CAD build for the part. Positions are in the model's coordinates, mm. Face numbers are marked on the shaded views. A direction names the side the tool comes from. Round coordinates to 2 decimals unless told otherwise and drop trailing zeros. Write each loop counter-clockwise with the first axis right and the second up, starting at its lowest first coordinate (ties: lowest second). Pieces come first, ordered by that corner, then holes. Notation, with made-up numbers: (63.5, 50.5) - (79.5, 50.5) arc R15 cw to (79.5, 63.5) - close; hole circle Ø11 at (46.5, 39). An arc over 180 degrees is marked (long way). Put each result on its own line as item: value. Start each with the question number.
Item 1: 3-axis set-ups, long thin cutter, end or side, ignore diameter. For the marked faces 1 and 2: which of +Z, -Z, +X, -X, +Y, -Y reach the whole face in a straight line?
Item 2: Cut at C-C (z = 41). Give the cut face in (x, y).
Item 3: Drill centre lines: line 1 (Z direction, x = 9.5, y = -7.75); line 2 (X direction, y = -0.25, z = 40.5); line 3 (Y direction, x = -0.5, z = 35.5). Where is each one in solid material? Low to high. Write a range as from..to.
Item 4: Cut at B-B (y = 0). Give the cut face in (x, z).
Item 5: Cut at A-A (x = 0). Give the cut face in (y, z).
Item 6: Pin check, flat tips, straight feed: pin 1 Ø5 at (x, y) = (-9.5, -0.5) entering from -Z; pin 2 Ø5 at (x, z) = (-7.5, 37) entering from +Y. Stop position of each tip, or through.
```python
from build123d import *

# Parameters (mm, degrees)
F0_W     = 29.464
F0_H     = 25.4508
F1_DEPTH = 50.9778
F2_W     = 39.90591
F2_H     = 36.580414
F2_R     = 12
F3_DEPTH = 19.05


with BuildPart() as f1:
    # F0 (on Top) → F1 (new body)
    with BuildSketch(Plane.XY):
        Rectangle(F0_W, F0_H)
    extrude(amount=F1_DEPTH)

    # F2 (on face) → F3 (cut)
    with BuildSketch(Plane.XY.offset(50.9778)):
        Rectangle(F2_W, F2_H)
        Circle(F2_R, mode=Mode.SUBTRACT)
    extrude(amount=-F3_DEPTH, mode=Mode.SUBTRACT)


solid = f1.part
```
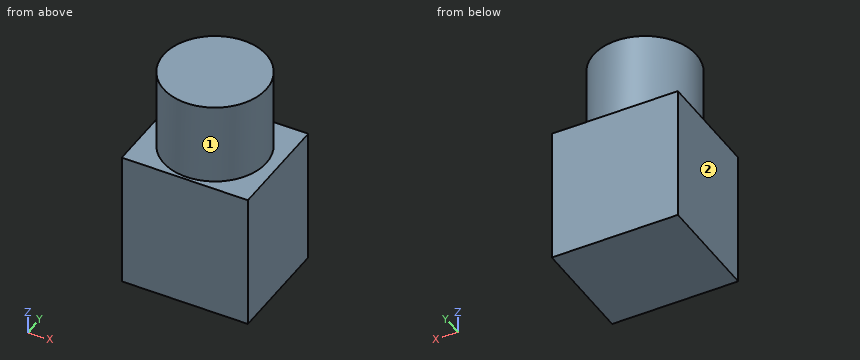
Output values:
1. face 1: +Z
1. face 2: +Z, -Z, -X, +Y, -Y
2. outline: circle Ø24 at (0, 0)
3. line 1: 0..31.93
3. line 2: -12..12
3. line 3: -11.99..11.99
4. outline: (-14.73, 0) - (14.73, 0) - (14.73, 31.93) - (12, 31.93) - (12, 50.98) - (-12, 50.98) - (-12, 31.93) - (-14.73, 31.93) - close
5. outline: (-12.73, 0) - (12.73, 0) - (12.73, 31.93) - (12, 31.93) - (12, 50.98) - (-12, 50.98) - (-12, 31.93) - (-12.73, 31.93) - close
6. pin 1: z = 0
6. pin 2: y = 10.91
